Verification items for the finished model (mm, model axes). Give positions to 0.01 mm unless a question says otherwise; leave off trailing zeros. Loops run counter-clockwise (first coordinate to the right, second up) from the corner with the lowest first, then second, coordinate; pieces in that order, holes last. Notation, with made-up numbers: (-22.75, 29) - (3.25, 29) arc R8 cw to (3.25, 35) - close; hole circle Ø2 at (-13, -36.75). An arc over 180 degrees is marked (long way). One line per item, written item: value. Start each with the question number.
1. Sectioned sample at C-C (x = 17.5). Record the cut outline in (y, z), plus the area to 3 significant figures.
2. Sectioned sample at B-B (z = 0.9). Record the cut outline in (x, y), plus the area to 3 significant figures.
3. Sectioned sample at D-D (x = 0). Record the cut outline in (y, z), plus the area to 3 significant figures.
4. Sectioned sample at A-A (y = 0.75). Record the cut outline in (x, z).
5. Scan lines: L1, parallel to Y at x = 18, z = 0.8; L2, parallel to Y at x = -2, z = 0.55; L3, parallel to X at y = -0.75, z = 1.2. Record each from-to range of solid material in increasing order. Write a range as [from, to].
Autodesk Inventor part; units mm, degrees
ref_plane "YZ Plane" through (0, 0, 0) normal (1, 0, 0) x (0, 1, 0)
ref_plane "XZ Plane" through (0, 0, 0) normal (0, 1, 0) x (-1, 0, 0)
ref_plane "XY Plane" through (0, 0, 0) normal (0, 0, 1) x (1, 0, 0)
sketch "スケッチ1" plane through (0, 0, 0) normal (0, 0, 1) x (1, 0, 0)
  circle A0 centre (-18, 0) radius 1.1
  circle A1 centre (18, 0) radius 1.1
  circle A2 centre (-18, 0) radius 2
  circle A3 centre (18, 0) radius 2
  line L0 (3, 7) -> (13, 7)
  line L1 (13, 7) -> (13, 4)
  line L2 (13, 4) -> (3, 4)
  line L3 (3, 4) -> (3, 7)
  circle A4 centre (4.1, 4) radius 1.1
  line L4 (8, 7) -> (8, 3.6941) construction
  circle A5 centre (11.9, 4) radius 1.1
  circle A6 centre (18, 5.5) radius 1.1
  circle A7 centre (-2, 5.5) radius 1.1
  circle A8 centre (-2, 5.5) radius 2
  circle A9 centre (18, 5.5) radius 2
  line L5 (-18.6502, 1.8914) -> (-2.6502, 7.3914)
  line L6 (-2, 7.5) -> (3, 7.5)
  line L7 (3, 7.5) -> (3, 7)
  line L8 (20, 5.5) -> (20, 0)
  line L9 (-18, -2) -> (18, -2)
  line L10 (18, 7.5) -> (13, 7.5)
  line L11 (13, 7.5) -> (13, 7)
  point P0 (0, 0)
  point P1 (13, 5.5)
  point P2 (10.8, 4)
  point P3 (5.2, 4)
  dimension "d0" = 2.2
  dimension "d1" = 2.2
  dimension "d2" = 36
  dimension "d3" = 18
  dimension "d4" = 4
  dimension "d5" = 4
  dimension "d6" = 3
  dimension "d7" = 10
  dimension "d8" = 2.2
  dimension "d9" = 2.2
  dimension "d10" = 5
  dimension "d11" = 4
  dimension "d12" = 4
  dimension "d13" = 4
extrude "押し出し1" add sketch "スケッチ1" along normal blind 1.5 contours A2 | A2 L5 A8 L6 L7 L3 A4 L2 A5 L1 L11 L10 A9 L8 A3 L9 | A8 | A3 | A9
sketch "スケッチ3" plane through (0, 0, 1.5) normal (0, 0, 1) x (1, 0, 0)
  circle A0 centre (11.5, -8) radius 8
  line L0 (-6.1786, -1.5714) -> (-6.1786, -5.4286)
  line L1 (0.1786, -1.5714) -> (-6.1786, -1.5714)
  line L2 (0.1786, -5.4286) -> (0.1786, -1.5714)
  line L3 (-18, -2) -> (18, -2)
  line L4 (-6.6786, -5.4286) -> (-6.6786, -1.0714)
  line L5 (-6.6786, -1.0714) -> (0.6786, -1.0714)
  line L6 (0.6786, -1.0714) -> (0.6786, -5.4286)
  point P0 (0, 0)
  point P1 (3.6112, -2)
  point P2 (0.6786, -2)
  point P3 (-6.6786, -2)
  dimension "d22" = 0.5
extrude "押し出し3" cut sketch "スケッチ3" against normal through all
fillet "フィレット2" radius 2 2 edges at (0.6786, -2, 0.75) (-6.6786, -2, 0.75)
equation "\"d12\" = d11"
properties part number "kosiyosetuzoku"
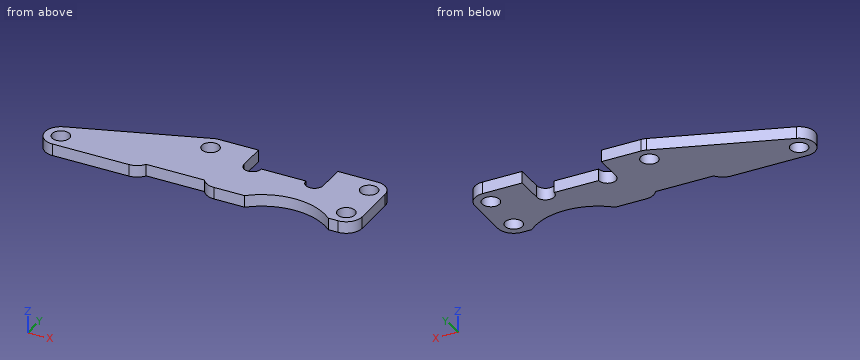
Results are:
1. outline: (-2, 0) - (-0.98, 0) - (-0.98, 1.5) - (-2, 1.5) - close; (0.98, 0) - (4.52, 0) - (4.52, 1.5) - (0.98, 1.5) - close; (6.48, 0) - (7.5, 0) - (7.5, 1.5) - (6.48, 1.5) - close
1. area: 8.37 mm^2
2. outline: (-18.65, 1.89) arc R2 ccw to (-18, -2) - (-8.37, -2) arc R2 ccw to (-6.68, -1.07) - (0.68, -1.07) arc R2 ccw to (2.37, -2) - (6.21, -2) arc R8 cw to (16.79, -2) - (18, -2) arc R2 ccw to (20, 0) - (20, 5.5) arc R2 ccw to (18, 7.5) - (13, 7.5) - (13, 4) arc R1.1 cw to (10.8, 4) - (5.2, 4) arc R1.1 cw to (3, 4) - (3, 7.5) - (-2, 7.5) arc R2 ccw to (-2.65, 7.39) - close; hole circle Ø2.2 at (-18, 0); hole circle Ø2.2 at (-2, 5.5); hole circle Ø2.2 at (18, 0); hole circle Ø2.2 at (18, 5.5)
2. area: 247 mm^2
3. outline: (-1.07, 0) - (7.5, 0) - (7.5, 1.5) - (-1.07, 1.5) - close
3. area: 12.9 mm^2
4. outline: (-19.85, 0) - (-18.8, 0) - (-18.8, 1.5) - (-19.85, 1.5) - close; (-17.2, 0) - (17.2, 0) - (17.2, 1.5) - (-17.2, 1.5) - close; (18.8, 0) - (20, 0) - (20, 1.5) - (18.8, 1.5) - close
5. L1: y = [-2, -1.1], [1.1, 4.4], [6.6, 7.5]
5. L2: y = [-1.07, 4.4], [6.6, 7.5]
5. L3: x = [-19.85, -18.8], [-17.2, 8.12], [14.88, 17.2], [18.8, 19.85]
